The model under review builds one solid part; all positions refer to its coordinate system, in mm. A direction names the side the tool comes from. Round coordinates to 2 decimals unless told otherwise and drop trailing zeros. Order: outer loops, then holes, each group sorted by start corner. A loop starts at its lowest first (then second) coordinate and runs counter-clockwise, first axis right, second up. Notation, with made-up numbers: (-14, 19.5) -> (12, 19.5) arc R24 ccw to (12, 42.5) -> close; hole circle Ø10 at (-36.5, 89). An arc over 180 degrees is marked (long way). Return JSON: item names as keys, results as strings. Group by question number.
from build123d import *

# Parameters (mm, degrees)
F0_R     = 228.6
F1_DEPTH = 19.05
F2_R     = 38.1
F3_DEPTH = 19.051
F4_R     = 4.7625
F4_R_2   = 3.302
F5_DEPTH = 19.051
F6_R     = 10.795
F6_R_2   = 9.525
F7_DEPTH = 6.35


# Not quite as in the source:
# - a fillet or chamfer that OpenCascade refuses, or shapes differently, is made with other operations: its cross-section is extruded or revolved along the edge and cut away or added


with BuildPart() as f1:
    # F0 (on Front) → F1 (new body)
    with BuildSketch(Plane.XZ):
        Circle(F0_R)
    extrude(amount=F1_DEPTH)

    # F2 (on face) → F3 (cut, through all)
    with BuildSketch(Plane.XZ.offset(19.05)):
        Circle(F2_R)
    extrude(amount=-F3_DEPTH, mode=Mode.SUBTRACT)

    # F4 (on face) → F5 (cut, through all)
    with BuildSketch(Plane.XZ.offset(19.05)):
        with Locations((107.7630734528, 107.7630734528)):
            Circle(F4_R)
        with Locations((125.723585695, 125.723585695)):
            Circle(F4_R)
        with Locations((-107.7630734528, 107.7630734528)):
            Circle(F4_R)
        with Locations((-125.723585695, 125.723585695)):
            Circle(F4_R)
        with Locations((-99.4616398417, -184.3144535841)):
            Circle(F4_R_2)
        with Locations((-184.3144535841, -99.4616398417)):
            Circle(F4_R_2)
        with Locations((99.4616398417, -184.3144535841)):
            Circle(F4_R_2)
        with Locations((184.3144535841, -99.4616398417)):
            Circle(F4_R_2)
    extrude(amount=-F5_DEPTH, mode=Mode.SUBTRACT)

    # F6 (on face) → F7 (cut)
    with BuildSketch(Plane.XZ.offset(19.05)):
        with Locations((107.7630734528, 107.7630734528)):
            Circle(F6_R)
        with Locations((125.723585695, 125.723585695)):
            Circle(F6_R)
        with Locations((-125.723585695, 125.723585695)):
            Circle(F6_R)
        with Locations((-107.7630734528, 107.7630734528)):
            Circle(F6_R)
        with Locations((-184.3144535841, -99.4616398417)):
            Circle(F6_R_2)
        with Locations((-99.4616398417, -184.3144535841)):
            Circle(F6_R_2)
        with Locations((99.4616398417, -184.3144535841)):
            Circle(F6_R_2)
        with Locations((184.3144535841, -99.4616398417)):
            Circle(F6_R_2)
    extrude(amount=-F7_DEPTH, mode=Mode.SUBTRACT)

    # F8: fillet of radius 12.7 on 2 edges, made by hand

    # F8_s1 → F8_t2 (revolve, cut)
    with BuildSketch(Plane.XY):
        with BuildLine():
            ThreePointArc((228.6, -6.35), (224.8802561211, -15.3302561211), (215.9, -19.05))
            Line((215.9, -19.05), (228.6, -19.05))
            Line((228.6, -19.05), (228.6, -6.35))
        make_face()
    revolve(axis=Axis((0, -19.05, 0), (0, -1, 0)), mode=Mode.SUBTRACT)

    # F8_s3 → F8_t4 (revolve, cut)
    with BuildSketch(Plane.XY):
        with BuildLine():
            ThreePointArc((50.8, -19.05), (41.8197438789, -15.3302561211), (38.1, -6.35))
            Line((38.1, -6.35), (38.1, -19.05))
            Line((38.1, -19.05), (50.8, -19.05))
        make_face()
    revolve(axis=Axis((0, -19.05, 0), (0, -1, 0)), mode=Mode.SUBTRACT)


solid = f1.part
Item 1: Consider section C-C on y = -9.25. Give the number of separate pieces and of enclosed holes in the cut face, plus the area to 3 significant figures.
Item 2: Consider section B-B on x = 0. State the section outline as (y, z) points, plus the area to 3 significant figures.
Item 3: Consider section A-A on z = 0. State the section outline as (x, y) points, plus the area to 3 significant figures.
Item 4: The part is to be moulded in two halves that separate along X. For faces 3 (the face through (-184, -12.7, -104)), 4 (the face through (-3, 0, -48)), say which applies: +X half, -X half, draft (parallel to the pull), parting line (faces both ways), or undercut.
Item 5: Insertion check: pin 1 Ø17.5 at (x, z) = (-125.72, 125.72) entering from -Y; pin 2 Ø3 at (y, z) = (-9, -16) entering from +X; pin 3 Ø10 at (y, z) = (-13.5, 138) entering from +X; pin 4 Ø8.5 at (x, z) = (107.76, 107.76) entering from +Y. Each pin has a flat end and moves straight along its axis. Give the tip position at first contact, or say it passes through.
Item 6: For faces 1 (the face through (188, -12.7, -99)), 2 (the face through (-3, -19.05, 51)), list the 3-axis set-ups (+Z, -Z, +X, -X, +Y, -Y) from which the entire face can be reached by the end or side of a thin tool; tool diameter is ignored.
Item 7: Wall thickness on line 1 along X through (y, z) = (-16.5, 130); line 2 along X through (y, z) = (-12.75, 128); line 3 along Z through (x, y) = (0, -2.25): over which ranges is each line inside the solid? List them lowest first.
Values:
{
 "1": {"separate pieces": "1", "enclosed holes": "9", "area": "159,000 mm^2"},
 "2": {"outline": "(-19.05, -215.9) arc R12.7 ccw to (-6.35, -228.6) -> (0, -228.6) -> (0, -38.1) -> (-6.35, -38.1) arc R12.7 ccw to (-19.05, -50.8) -> close; (-19.05, 50.8) arc R12.7 ccw to (-6.35, 38.1) -> (0, 38.1) -> (0, 228.6) -> (-6.35, 228.6) arc R12.7 ccw to (-19.05, 215.9) -> close", "area": "7,120 mm^2"},
 "3": {"outline": "(-228.6, -6.35) arc R12.7 ccw to (-215.9, -19.05) -> (-50.8, -19.05) arc R12.7 ccw to (-38.1, -6.35) -> (-38.1, 0) -> (-228.6, 0) -> close; (38.1, -6.35) arc R12.7 ccw to (50.8, -19.05) -> (215.9, -19.05) arc R12.7 ccw to (228.6, -6.35) -> (228.6, 0) -> (38.1, 0) -> close", "area": "7,120 mm^2"},
 "4": {"face 3": "undercut", "face 4": "draft"},
 "5": {"pin 1": "y = -12.7", "pin 2": "x = 228.02", "pin 3": "x = 184.36", "pin 4": "through"},
 "6": {"face 1": "-Y", "face 2": "+Z, -Z, +X, -X, -Y"},
 "7": {"line 1": "-181.84 to -135.64, -115.81 to 115.81, 135.64 to 181.84", "line 2": "-187.31 to -136.28, -115.17 to 115.17, 136.28 to 187.31", "line 3": "-228.6 to -38.1, 38.1 to 228.6"}
}
